Work out the finished part from the listing and answer in its coordinate system (mm). A direction names the side the tool comes from. Coordinates: 2 decimals unless noted, no trailing zeros. Order: outer loops, then holes, each group sorted by start corner. A loop starts at its lowest first (then second) coordinate and runs counter-clockwise, first axis right, second up. Notation, with made-up numbers: M 88,76.5 L 136,76.5 A13 ccw 136,88.5 Z; hole C 40,76 d10. An arc over 180 degrees is marked long. Use a Markdown table: item, result. Add a question column.
from build123d import *

# Parameters (mm, degrees)
EXTRUDE_1_DEPTH        = 21
CUT_EXTRUDE_1_REACH    = 67.376
CUT_EXTRUDE_2_REACH    = 67.376
SKETCH_3_R             = 4
SKETCH_3_R_2           = 1
SKETCH_4_R             = 4
SKETCH_4_R_2           = 1.026612686
SKETCH_4_R_3           = 1
CUT_EXTRUDE_3_DEPTH    = 1
SKETCH_6_W             = 49
SKETCH_6_H             = 1
EXTRUDE_2_DEPTH        = 1
SKETCH_7_W             = 49
SKETCH_7_H             = 1
EXTRUDE_3_DEPTH        = 3
FILLET_1_R             = 2
FILLET_1_OF_MIRROR_3_R = 2
EXTRUDE_START          = -1
EXTRUDE_4_DEPTH        = 1
SKETCH_10_W            = 1
SKETCH_10_H            = 1
EXTRUDE_5_DEPTH        = 1


with BuildPart() as part:
    # 草图1 → 凸台-拉伸1 (new body)
    with BuildSketch(Plane.XY):
        Polygon((-26.5, 1), (-26.5, -32), (-25.5, -32), (-25.5, 0), (25.5, 0), (25.5, -32), (26.5, -32), (26.5, 1), align=None)
    extrude(amount=EXTRUDE_1_DEPTH)

    # 切除-拉伸1: up to this face of the body (flat: up to its plane)
    cut_extrude_1_end = Plane(part.part.faces().sort_by_distance((26.5, -15.5, 10.5))[0])
    # 草图2 → 切除-拉伸1 (cut, up to the picked face)
    with BuildSketch(Plane.ZY.offset(26.5), mode=Mode.PRIVATE) as cut_extrude_1_sk1:
        with BuildLine():
            Line((0, -32), (10.5, -32))
            ThreePointArc((10.5, -32), (3.075378798, -28.924621202), (0, -21.5))
            Line((0, -21.5), (0, -32))
        make_face()
    cut_extrude_1_tool1 = split(extrude(cut_extrude_1_sk1.sketch, amount=-CUT_EXTRUDE_1_REACH, mode=Mode.PRIVATE), bisect_by=cut_extrude_1_end, keep=Keep.BOTH, mode=Mode.PRIVATE)
    cut_extrude_1 = cut_extrude_1_tool1.solids().sort_by(Axis((-26.5, -29.654637, 2.345363), (1, 0, 0)))[0]
    add(cut_extrude_1, mode=Mode.SUBTRACT)

    # 镜向1: 切除-拉伸1 across plane
    add(cut_extrude_1.mirror(Plane.XY.offset(10.5)), mode=Mode.SUBTRACT)

    # 切除-拉伸2: up to this face of the body (flat: up to its plane)
    cut_extrude_2_end = Plane(part.part.faces().sort_by_distance((-26.5, -14.462654994, 10.5))[0])
    # 草图3 → 切除-拉伸2 (cut, up to the picked face)
    with BuildSketch(Plane(origin=(26.5, 0, 0), x_dir=(0, 0, -1), z_dir=(1, 0, 0)), mode=Mode.PRIVATE) as cut_extrude_2_sk1:
        with Locations(Location((-10.5, -22, 0), (0, 0, 90))):
            Circle(SKETCH_3_R)
    cut_extrude_2_tool1 = split(extrude(cut_extrude_2_sk1.sketch, amount=-CUT_EXTRUDE_2_REACH, mode=Mode.PRIVATE), bisect_by=cut_extrude_2_end, keep=Keep.BOTH, mode=Mode.PRIVATE)
    # 草图3 → 切除-拉伸2 (cut, up to the picked face)
    with BuildSketch(Plane(origin=(26.5, 0, 0), x_dir=(0, 0, -1), z_dir=(1, 0, 0)), mode=Mode.PRIVATE) as cut_extrude_2_sk2:
        with Locations(Location((-3.5, -22, 0), (0, 0, 90))):
            Circle(SKETCH_3_R_2)
    cut_extrude_2_tool2 = split(extrude(cut_extrude_2_sk2.sketch, amount=-CUT_EXTRUDE_2_REACH, mode=Mode.PRIVATE), bisect_by=cut_extrude_2_end, keep=Keep.BOTH, mode=Mode.PRIVATE)
    # 草图3 → 切除-拉伸2 (cut, up to the picked face)
    with BuildSketch(Plane(origin=(26.5, 0, 0), x_dir=(0, 0, -1), z_dir=(1, 0, 0)), mode=Mode.PRIVATE) as cut_extrude_2_sk3:
        with Locations(Location((-10.5, -15, 0), (0, 0, 90))):
            Circle(SKETCH_3_R_2)
    cut_extrude_2_tool3 = split(extrude(cut_extrude_2_sk3.sketch, amount=-CUT_EXTRUDE_2_REACH, mode=Mode.PRIVATE), bisect_by=cut_extrude_2_end, keep=Keep.BOTH, mode=Mode.PRIVATE)
    # 草图3 → 切除-拉伸2 (cut, up to the picked face)
    with BuildSketch(Plane(origin=(26.5, 0, 0), x_dir=(0, 0, -1), z_dir=(1, 0, 0)), mode=Mode.PRIVATE) as cut_extrude_2_sk4:
        with Locations(Location((-17.5, -22, 0), (0, 0, 90))):
            Circle(SKETCH_3_R_2)
    cut_extrude_2_tool4 = split(extrude(cut_extrude_2_sk4.sketch, amount=-CUT_EXTRUDE_2_REACH, mode=Mode.PRIVATE), bisect_by=cut_extrude_2_end, keep=Keep.BOTH, mode=Mode.PRIVATE)
    # 草图3 → 切除-拉伸2 (cut, up to the picked face)
    with BuildSketch(Plane(origin=(26.5, 0, 0), x_dir=(0, 0, -1), z_dir=(1, 0, 0)), mode=Mode.PRIVATE) as cut_extrude_2_sk5:
        with Locations(Location((-10.5, -29, 0), (0, 0, 90))):
            Circle(SKETCH_3_R_2)
    cut_extrude_2_tool5 = split(extrude(cut_extrude_2_sk5.sketch, amount=-CUT_EXTRUDE_2_REACH, mode=Mode.PRIVATE), bisect_by=cut_extrude_2_end, keep=Keep.BOTH, mode=Mode.PRIVATE)
    add(cut_extrude_2_tool1.solids().sort_by(Axis((26.5, -22, 10.5), (-1, 0, 0)))[0], mode=Mode.SUBTRACT)
    add(cut_extrude_2_tool2.solids().sort_by(Axis((26.5, -22, 3.5), (-1, 0, 0)))[0], mode=Mode.SUBTRACT)
    add(cut_extrude_2_tool3.solids().sort_by(Axis((26.5, -15, 10.5), (-1, 0, 0)))[0], mode=Mode.SUBTRACT)
    add(cut_extrude_2_tool4.solids().sort_by(Axis((26.5, -22, 17.5), (-1, 0, 0)))[0], mode=Mode.SUBTRACT)
    add(cut_extrude_2_tool5.solids().sort_by(Axis((26.5, -29, 10.5), (-1, 0, 0)))[0], mode=Mode.SUBTRACT)

    # 草图4 → 切除-拉伸3 (cut)
    with BuildSketch(Plane(origin=(0, 1, 0), x_dir=(1, 0, 0), z_dir=(0, 1, 0))):
        with Locations(Location((0, -10.5, 0), (0, 0, 180))):
            Circle(SKETCH_4_R)
        with Locations(Location((5, -5.5, 0), (0, 0, 180))):
            Circle(SKETCH_4_R_2)
        with Locations(Location((13.5, -10.5, 0), (0, 0, 180))):
            Circle(SKETCH_4_R_3)
        with Locations(Location((-13.5, -10.5, 0), (0, 0, 180))):
            Circle(SKETCH_4_R_3)
        with Locations((5, -15.5)):
            Circle(SKETCH_4_R_2)
        with Locations((-5, -5.5)):
            Circle(SKETCH_4_R_2)
        with Locations(Location((-5, -15.5, 0), (0, 0, 180))):
            Circle(SKETCH_4_R_2)
    extrude(amount=-CUT_EXTRUDE_3_DEPTH, mode=Mode.SUBTRACT)

    # 草图6 → 凸台-拉伸2 (add)
    with BuildSketch(Plane.XY.offset(21)):
        with Locations((0, 0.5)):
            Rectangle(SKETCH_6_W, SKETCH_6_H)
    extrude_2 = extrude(amount=EXTRUDE_2_DEPTH)

    # 草图7 → 凸台-拉伸3 (add)
    with BuildSketch(Plane.XZ):
        with Locations((0, 21.5)):
            Rectangle(SKETCH_7_W, SKETCH_7_H)
    extrude_3 = extrude(amount=EXTRUDE_3_DEPTH)

    # 圆角1
    fillet_1_edges = [part.edges().sort_by_distance(p)[0] for p in [
        (24.5, -3, 21.5),
        (-24.5, -3, 21.5),
    ]]
    fillet(fillet_1_edges, radius=FILLET_1_R)

    # 镜向3: 凸台-拉伸2, 凸台-拉伸3 across plane
    add(extrude_2.mirror(Plane.XY.offset(10.5)))
    add(extrude_3.mirror(Plane.XY.offset(10.5)))

    # 圆角1 of 镜向3
    fillet_1_of_mirror_3_edges = [part.edges().sort_by_distance(p)[0] for p in [
        (24.5, -3, -0.5),
        (-24.5, -3, -0.5),
    ]]
    fillet(fillet_1_of_mirror_3_edges, radius=FILLET_1_OF_MIRROR_3_R)

    # 草图9 → 凸台-拉伸4 (add)
    with BuildSketch(Plane(origin=(26.5, 0, 0), x_dir=(0, 0, -1), z_dir=(1, 0, 0)).offset(EXTRUDE_START)):
        with BuildLine():
            Line((-21, 1), (-22, 1))
            Line((-22, 1), (-22, -21.5))
            ThreePointArc((-22, -21.5), (-10.5, -33), (1, -21.5))
            Line((1, -21.5), (1, 1))
            Line((1, 1), (0, 1))
            Line((0, 1), (0, -21.5))
            ThreePointArc((0, -21.5), (-10.5, -32), (-21, -21.5))
            Line((-21, -21.5), (-21, 1))
        make_face()
    extrude_4 = extrude(amount=EXTRUDE_4_DEPTH)

    # 镜向4: 凸台-拉伸4 across plane
    add(extrude_4.mirror(Plane(origin=(0, 0, 0), x_dir=(0, 0, 1), z_dir=(1, 0, 0))))

    # 草图10 → 凸台-拉伸5 (add)
    with BuildSketch(Plane(origin=(0, 1, 0), x_dir=(1, 0, 0), z_dir=(0, 1, 0))):
        with Locations((-25, 0.5)):
            Rectangle(SKETCH_10_W, SKETCH_10_H)
        with Locations((-25, -21.5)):
            Rectangle(SKETCH_10_W, SKETCH_10_H)
        with Locations((25, 0.5)):
            Rectangle(SKETCH_10_W, SKETCH_10_H)
        with Locations((25, -21.5)):
            Rectangle(SKETCH_10_W, SKETCH_10_H)
    extrude(amount=-EXTRUDE_5_DEPTH)


solid = part.part
(1) A cutting plane is placed at B-B on x = -5. Write down the section's boundary in (y, z), plus the area to 3 significant figures.
(2) Given P1, Ø2.5, axis at x = 5, z = 5.5, coming from the -Y side; P2, Ø1.8, axis at x = -5, z = 5.5, coming from the +Y side (1 decimal); P3, Ø0.8, axis at x = 1, z = -0.5, coming from the -Y side, each flat-ended and moving along its own axis, determine where each tip first touches the part or whether it passes through.
(3) A cutting plane is placed at C-C on y = -9. Write down the section's boundary in (x, z), plus the area to 3 significant figures.
(4) A cutting plane is placed at A-A on y = -15. Write down the section's boundary in (x, z), plus the area to 3 significant figures.
(5) A cutting plane is placed at D-D on x = 13.5. Write down the section's boundary in (y, z), plus the area to 3 significant figures.
(6) The mould has two halves that part along Z. Classify faces 1 (the cylindrical face through (-4.24, 0.51, 16.19)), 2 (the flat face through (-26.5, -12, 11)), 3 (the flat face through (4, -2, 22)), 4 (the cylindrical face through (-25.993, -32.997, 10.753)): pulls with the +Z half, pulls with the -Z half, needs draft (parallel to the pull), parting line crosses it, or undercut.
(7) Straight lines are drawn through the part: line 1 (Z direction, x = 26, y = -22); line 2 (Z direction, x = -26.25, y = -15); line 3 (X direction, y = -23, z = 15). For each, find the intervals that lie inside material, in ascending order.
(8) Which of the six approach directions +Z, -Z, +X, -X, +Y, -Y give full straight-line access (tool end or side, diameter ignored) to faces 5 (the cylindrical face through (5.13, 0.51, 6.52)), 6 (the flat face through (0, -1, 21)), 7 (the cylindrical face through (-23.93, -2.4, -0.51))?
From the geometry:
| question | item | result |
|---|---|---|
| 1 | outline | M -3,-1 L 1,-1 L 1,4.47 L 0,4.47 L 0,0 L -3,0 Z; M -3,21 L 0,21 L 0,16.53 L 1,16.53 L 1,22 L -3,22 Z; M 0,6.53 L 1,6.53 L 1,14.47 L 0,14.47 Z |
| 1 | area | 24.9 mm2 |
| 2 | P1 | stops at y = 0 |
| 2 | P2 | passes through |
| 2 | P3 | stops at y = -3 |
| 3 | outline | M -26.5,-1 L -25.5,-1 L -25.5,22 L -26.5,22 Z; M 25.5,-1 L 26.5,-1 L 26.5,22 L 25.5,22 Z |
| 3 | area | 46.0 mm2 |
| 4 | outline | M -26.5,-1 L -25.5,-1 L -25.5,9.5 L -26.5,9.5 Z; M -26.5,11.5 L -25.5,11.5 L -25.5,22 L -26.5,22 Z; M 25.5,-1 L 26.5,-1 L 26.5,9.5 L 25.5,9.5 Z; M 25.5,11.5 L 26.5,11.5 L 26.5,22 L 25.5,22 Z |
| 4 | area | 42.0 mm2 |
| 5 | outline | M -3,-1 L 1,-1 L 1,9.5 L 0,9.5 L 0,0 L -3,0 Z; M -3,21 L 0,21 L 0,11.5 L 1,11.5 L 1,22 L -3,22 Z |
| 5 | area | 27.0 mm2 |
| 6 | face 1 | undercut |
| 6 | face 2 | needs draft |
| 6 | face 3 | pulls with the +Z half |
| 6 | face 4 | parting line crosses it |
| 7 | line 1 | z = -0.99 to 2.5, 4.5 to 6.5, 14.5 to 16.5, 18.5 to 21.99 |
| 7 | line 2 | z = -1 to 9.5, 11.5 to 22 |
| 7 | line 3 | x = -26.5 to -25.5, 25.5 to 26.5 |
| 8 | face 5 | +Y, -Y |
| 8 | face 6 | -Y |
| 8 | face 7 | +Z, -Z, -Y |
